The model under review builds one solid part; all positions refer to its coordinate system, in mm. Face numbers are marked on the shaded views. A direction names the side the tool comes from. Round coordinates to 2 decimals unless told otherwise and drop trailing zeros. Write each loop counter-clockwise with the first axis right and the second up, starting at its lowest first coordinate (ties: lowest second). Pieces come first, ordered by that corner, then holes. Notation, with made-up numbers: (25.5, 21.25) -> (65.5, 21.25) arc R27 cw to (65.5, 52.25) -> close; hole circle Ø3 at (-7.5, 23.25). An arc over 180 degrees is marked (long way). Return JSON: item names as keys, results as strings. Group by question number.
1. Take a section at D-D, the plane y = 22. Write out the cut boundary in (x, z).
2. Take a section at A-A, the plane z = 11.5. Write out the cut boundary in (x, y).
3. Take a section at B-B, the plane y = 48.5. Write out the cut boundary in (x, z), then the cut area to 3 significant figures.
4. For line 1 along X through (y, z) = (53.5, 26.5); line 2 along Z through (x, y) = (-115, 72); line 3 along Y through (x, z) = (-128, 9.25), list the stretches that pass through material, from the lowest coordinate up. Write a range as from..to.
5. Clearance check with flat-ended pins moving along their axes: P1, Ø12, axis at x = -131.5, z = 17.5, coming from the -Y side; P2, Ø16, axis at y = 43, z = 19.5, coming from the -X side; P3, Ø7, axis at x = -104, y = 48, coming from the +Z side. State where each tip first meets the part, or that it passes through.
6. Take a section at C-C, the plane x = -104. Write out the cut boundary in (y, z), then the cut area to 3 significant figures.
7. Mouldability with a two-part tool opening along X and no side actions: class the marked faces 3, 4, 5 and 6 as pulls with the +X half, pulls with the -X half, needs draft (parallel to the pull), parting line crosses it, or undercut.
8. Tool access review of the marked faces 1 and 2: name each direction out of +Z, -Z, +X, -X, +Y, -Y from which nothing blocks a thin tool from reaching the whole face with its end or side.
from build123d import *

# Parameters (mm, degrees)
ESQUISSE1_W        = 169
ESQUISSE1_H        = 82
BOSS_EXTRU_1_DEPTH = 9
ESQUISSE2_W        = 10
ESQUISSE2_H        = 30
BOSS_EXTRU_2_DEPTH = 82
ESQUISSE3_W        = 80
ESQUISSE3_H        = 4
BOSS_EXTRU_4_DEPTH = 20
ESQUISSE4_W        = 4
ESQUISSE4_H        = 20
BOSS_EXTRU_5_DEPTH = 20
ESQUISSE5_W        = 4
ESQUISSE5_H        = 20
BOSS_EXTRU_6_DEPTH = 20
ESQUISSE6_W        = 72
ESQUISSE6_H        = 3
BOSS_EXTRU_7_DEPTH = 5


with BuildPart() as part:
    # Esquisse1 → Boss.-Extru.1 (new body)
    with BuildSketch(Plane.XY):
        with Locations((-84.5, 41)):
            Rectangle(ESQUISSE1_W, ESQUISSE1_H)
    extrude(amount=BOSS_EXTRU_1_DEPTH)

    # Esquisse2 → Boss.-Extru.2 (add)
    with BuildSketch(Plane(origin=(0, 82, 0), x_dir=(1, 0, 0), z_dir=(0, 1, 0))):
        with Locations((5, -15)):
            Rectangle(ESQUISSE2_W, ESQUISSE2_H)
    extrude(amount=-BOSS_EXTRU_2_DEPTH)

    # Esquisse3 → Boss.-Extru.4 (add)
    with BuildSketch(Plane.XY.offset(9)):
        with Locations((-90, 34)):
            Rectangle(ESQUISSE3_W, ESQUISSE3_H)
    extrude(amount=BOSS_EXTRU_4_DEPTH)

    # Esquisse4 → Boss.-Extru.5 (add)
    with BuildSketch(Plane(origin=(0, 36, 0), x_dir=(1, 0, 0), z_dir=(0, 1, 0))):
        with Locations((-52, -19)):
            Rectangle(ESQUISSE4_W, ESQUISSE4_H)
    extrude(amount=BOSS_EXTRU_5_DEPTH)

    # Esquisse5 → Boss.-Extru.6 (add)
    with BuildSketch(Plane(origin=(0, 36, 0), x_dir=(1, 0, 0), z_dir=(0, 1, 0))):
        with Locations((-128, -19)):
            Rectangle(ESQUISSE5_W, ESQUISSE5_H)
    extrude(amount=BOSS_EXTRU_6_DEPTH)

    # Esquisse6 → Boss.-Extru.7 (add)
    with BuildSketch(Plane(origin=(0, 36, 0), x_dir=(1, 0, 0), z_dir=(0, 1, 0))):
        with Locations((-90, -27.5)):
            Rectangle(ESQUISSE6_W, ESQUISSE6_H)
    extrude(amount=BOSS_EXTRU_7_DEPTH)


solid = part.part
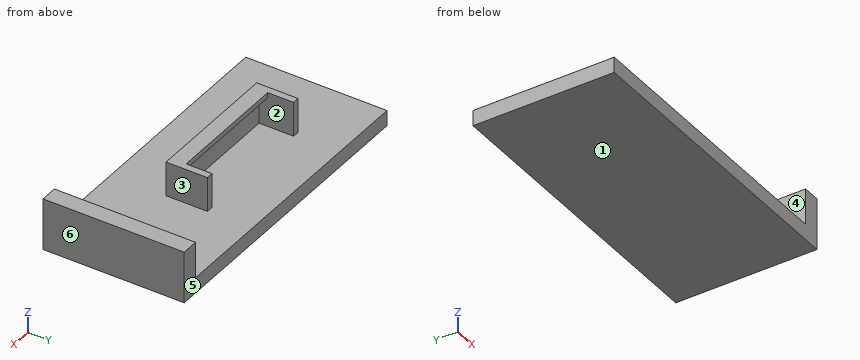
Output:
{
 "1": {"outline": "(-169, 0) -> (10, 0) -> (10, 30) -> (0, 30) -> (0, 9) -> (-169, 9) -> close"},
 "2": {"outline": "(-130, 32) -> (-50, 32) -> (-50, 56) -> (-54, 56) -> (-54, 36) -> (-126, 36) -> (-126, 56) -> (-130, 56) -> close; (0, 0) -> (10, 0) -> (10, 82) -> (0, 82) -> close"},
 "3": {"outline": "(-169, 0) -> (10, 0) -> (10, 30) -> (0, 30) -> (0, 9) -> (-50, 9) -> (-50, 29) -> (-54, 29) -> (-54, 9) -> (-126, 9) -> (-126, 29) -> (-130, 29) -> (-130, 9) -> (-169, 9) -> close", "area": "1,980 mm^2"},
 "4": {"line 1": "x = -130..-126, -54..-50, 0..10", "line 2": "z = 0..9", "line 3": "y = 32..56"},
 "5": {"P1": "stops at y = 32", "P2": "stops at x = -130", "P3": "stops at z = 9"},
 "6": {"outline": "(0, 0) -> (82, 0) -> (82, 9) -> (36, 9) -> (36, 26) -> (41, 26) -> (41, 29) -> (32, 29) -> (32, 9) -> (0, 9) -> close", "area": "833 mm^2"},
 "7": {"face 3": "undercut", "face 4": "undercut", "face 5": "needs draft", "face 6": "pulls with the +X half"},
 "8": {"face 1": "-Z, +X, -X, +Y, -Y", "face 2": "+Y"}
}
